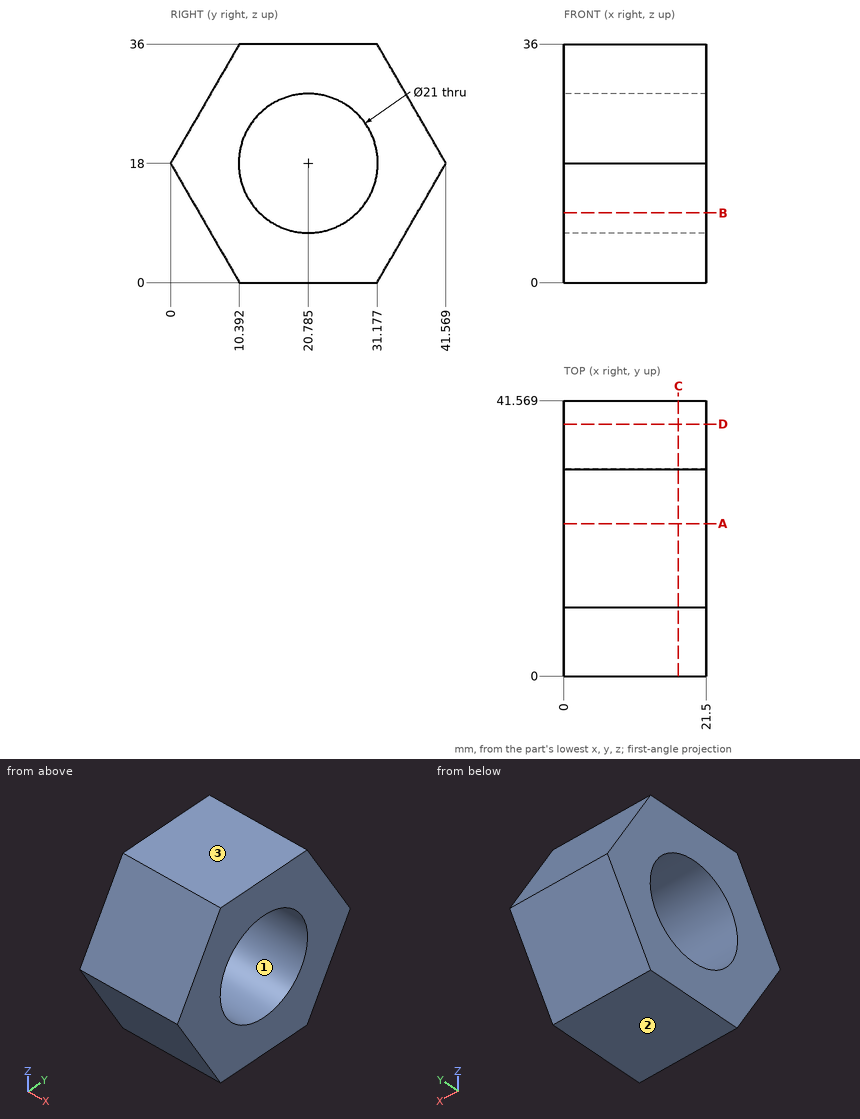
Geometry: see drawing. Coordinates: mm, zero at the bounding-box minimum. Round coordinates to 2 decimals unless told otherwise and drop trailing zeros. Order: outer loops, then holes, each group sorted by start corner. A loop starts at its lowest first (then second) coordinate and runs counter-clockwise, first axis right, second up. Notation, with made-up numbers: (38, 88) - (79, 88) arc R8 cw to (79, 96) - close; hole circle Ø10 at (-38.5, 25.25). An arc over 180 degrees is marked (long way). One line per question, with ' | ' between items. Start each with the question number.
1) Ray query, probe 1 along Y at (x, z) = (18.5, 15); probe 2 along Y at (x, z) = (4.25, 24) (1 decimal); probe 3 along Z at (x, y) = (1.75, 21.5) (1 decimal). Return the intervals inside material, ascending.
2) Cut plane B-B, the plane z = 10.5. Return the cut outline in (x, y).
3) Contact query for flat-ended pins moving along their axis: P1, Ø1.5, axis at x = 12, z = 24, coming from the -Y side; P2, Ø5, axis at y = 21, z = 10.5, coming from the -X side; P3, Ø4, axis at x = 12.5, z = 14.5, coming from the -Y side (1 decimal); P4, Ø5, axis at x = 3.5, z = 18.5, coming from the +Y side. Output: stop coordinate, or through.
4) Cut plane C-C, the plane x = 17.25. Return the cut outline in (y, z) (1 decimal), then the cut area to 3 significant figures.
5) Cut plane D-D, the plane y = 38. Return the cut outline in (x, z), then the cut area to 3 significant figures.
6) Cut plane A-A, the plane y = 23. Return the cut outline in (x, z), then the cut area to 3 significant figures.
7) Pull-direction query (Z, two-part tool) for the marked faces 1, 2 and 3; classes: +Z half, -Z half, draft (parallel to the pull), parting line (faces both ways), or undercut.
Worked out:
1) probe 1: y = 1.73 to 10.72, 30.85 to 39.84 | probe 2: y = 3.5 to 12.2, 29.4 to 38.1 | probe 3: z = 0 to 7.5, 28.5 to 36
2) outline: (0, 4.33) - (21.5, 4.33) - (21.5, 13.44) - (0, 13.44) - close; (0, 28.13) - (21.5, 28.13) - (21.5, 37.24) - (0, 37.24) - close
3) P1: stops at y = 3.03 | P2: passes through | P3: stops at y = 0.9 | P4: stops at y = 41.57
4) outline: (0, 18) - (10.4, 0) - (31.2, 0) - (41.6, 18) - (31.2, 36) - (10.4, 36) - close; hole circle Ø21 at (20.8, 18) | area: 776 mm^2
5) outline: (0, 11.82) - (21.5, 11.82) - (21.5, 24.18) - (0, 24.18) - close | area: 266 mm^2
6) outline: (0, 0) - (21.5, 0) - (21.5, 7.74) - (0, 7.74) - close; (0, 28.26) - (21.5, 28.26) - (21.5, 36) - (0, 36) - close | area: 333 mm^2
7) face 1: undercut | face 2: -Z half | face 3: +Z half
